```python
from build123d import *

# Parameters (mm, degrees)
CHAMFER_1_SIZE = 0.8


with BuildPart() as part:
    # Эскиз1 → Повернуть1 (revolve)
    with BuildSketch(Plane.XY, mode=Mode.PRIVATE) as revolve_1_sk:
        Polygon((0, 0), (-8.35, 0), (-8.35, -13), (-7.5, -13), (-7.5, -10.7), (-2.5, -10.7), (-2.5, -3), (0, -3), align=None)
    revolve(revolve_1_sk.sketch.rotate(Axis((0, -3, 0), (0, 1, 0)), 270), axis=Axis((0, -3, 0), (0, 1, 0)))

    # Фаска1
    chamfer_1_edges = [part.edges().sort_by_distance(p)[0] for p in [
        (0, 0, 8.35),
    ]]
    chamfer(chamfer_1_edges, length=CHAMFER_1_SIZE)


solid = part.part
```
For this review, take the finished solid that the model builds, in its own axes (mm). A direction names the side the tool comes from. Round coordinates to 2 decimals unless told otherwise and drop trailing zeros. Write each loop counter-clockwise with the first axis right and the second up, starting at its lowest first coordinate (ties: lowest second). Pieces come first, ordered by that corner, then holes. Notation, with made-up numbers: (29, -38.5) -> (73, -38.5) arc R19 cw to (73, -13.5) -> close; hole circle Ø4 at (5, -17.75). An arc over 180 degrees is marked (long way). One line per question, with ' | ' between items. Start each with the question number.
1) Wall thickness on line 1 along X through (y, z) = (-8.75, 0); line 2 along X through (y, z) = (-12.5, 0); line 3 along Y through (x, z) = (-4.5, 1.5): over which ranges is each line inside the solid? List them lowest first.
2) Mouldability with a two-part tool opening along Z and no side actions: class faces 1 (the cylindrical face through (-2.508, -6.985, -7.964)), 2 (the cylindrical face through (2.44, -6.8, 0.54)), 3 (the cylindrical face through (-0.33, -11.834, 7.493)), 4 (the flat face through (0, 0, 0)) as +Z half, -Z half, draft (parallel to the pull), parting line (faces both ways), or undercut.
3) Add section D-D (y = -1.25). Write out the cut boundary in (x, z).
4) Add section A-A (z = 0). Write out the cut boundary in (x, y).
5) Add section C-C (y = -9.5). Write out the cut boundary in (x, z).
6) Add section B-B (x = 0). Write out the cut boundary in (y, z).
7) Machinability: for faces 5 (the flat face through (0, -3, 0)), 6 (the flat face through (-5, -13, 6)), which of the approach directions +Z, -Z, +X, -X, +Y, -Y give a long, thin tool a straight path to every point of the face, cutting with its end or side? Answer none if there is none.
8) For pin 1 Ø1 at (x, z) = (5.5, -6.5) entering from +Y; pin 2 Ø4 at (y, z) = (-3.5, 5) entering from +X; pin 3 Ø1.5 at (y, z) = (-1.5, 5.5) entering from +X, all flat-tipped, find the tip position at first contact; note any pin that passes through.
Reported:
1) line 1: x = -8.35 to -2.5, 2.5 to 8.35 | line 2: x = -8.35 to -7.5, 7.5 to 8.35 | line 3: y = -10.7 to 0
2) face 1: parting line | face 2: undercut | face 3: undercut | face 4: draft
3) outline: circle Ø16.7 at (0, 0)
4) outline: (-8.35, -13) -> (-7.5, -13) -> (-7.5, -10.7) -> (-2.5, -10.7) -> (-2.5, -3) -> (2.5, -3) -> (2.5, -10.7) -> (7.5, -10.7) -> (7.5, -13) -> (8.35, -13) -> (8.35, -0.8) -> (7.55, 0) -> (-7.55, 0) -> (-8.35, -0.8) -> close
5) outline: circle Ø16.7 at (0, 0); hole circle Ø5 at (0, 0)
6) outline: (-13, -8.35) -> (-0.8, -8.35) -> (0, -7.55) -> (0, 7.55) -> (-0.8, 8.35) -> (-13, 8.35) -> (-13, 7.5) -> (-10.7, 7.5) -> (-10.7, 2.5) -> (-3, 2.5) -> (-3, -2.5) -> (-10.7, -2.5) -> (-10.7, -7.5) -> (-13, -7.5) -> close
7) face 5: -Y | face 6: +Z, -Z, +X, -X, -Y
8) pin 1: stops at y = -0.46 | pin 2: stops at x = 7.79 | pin 3: stops at x = 6.87
